Model file for the job. Use its own axes, mm. A direction names the side the tool comes from. Coordinates: 2 decimals unless noted, no trailing zeros. Order: outer loops, then holes, each group sorted by start corner. A loop starts at its lowest first (then second) coordinate and runs counter-clockwise, first axis right, second up. Notation, with made-up numbers: (-26, 87.25) -> (33, 87.25) arc R34 ccw to (33, 121.25) -> close; hole circle Ø7 at (73.5, 84). An arc over 180 degrees is marked (long way). Return JSON: item names as keys, results as strings. Group by question number.
1) Probe line 1 (X direction, y = 3.5, z = 22); line 2 (Z direction, x = -8.25, y = -1.5); line 3 (X direction, y = 3, z = 45.5). List the from-to ranges inside material, lowest first.
2) Cut at A-A (x = -14.75). Write the cut outline in (y, z) (3 decimals).
3) Flat gauge pins, fed straight in: pin 1 (3 mm diameter, centred on y = 2, z = 11.5, fed in from -X); pin 2 (1.8 mm diameter, centred on x = -15.32, z = 44.54, fed in from -Y); pin 3 (1.5 mm diameter, centred on y = 3, z = 33, fed in from +X); pin 4 (1.5 mm diameter, centred on x = -5.5, y = -2.5, fed in from +Z). Where does each tip first touch, or does it go through?
4) Pull direction Z, two halves, no side cores. Call faces 3 (the cylindrical face through (-0.56, -0.06, 2.72)), 4 (the cylindrical face through (-0.69, -0.06, 0.49)), 5 (the flat face through (-7, 4.5, 25)), 6 (the flat face through (-5.845, -0.063, 36.124)): +Z half, -Z half, draft (parallel to the pull), parting line (faces both ways), or undercut.
5) Cut at C-C (z = 45.5). Write the cut outline in (x, y), and give its area (3 significant figures).
6) Cut at D-D (z = 18.5). Write the cut outline in (x, y).
7) Cut at B-B (y = 3.5). Write the cut outline in (x, z), and give its area (3 significant figures).
8) Which spindle directions (+Z, -Z, +X, -X, +Y, -Y) get a long thin tool onto all of the face, cutting with end or side? Do faces 1 (the flat face through (-4, 0, 0)), 2 (the flat face through (-8, 0, 13)). Say none if no direction does.
Autodesk Inventor part; units mm, degrees
ref_plane "YZ Plane" through (0, 0, 0) normal (1, 0, 0) x (0, 1, 0)
ref_plane "XZ Plane" through (0, 0, 0) normal (0, 1, 0) x (-1, 0, 0)
ref_plane "XY Plane" through (0, 0, 0) normal (0, 0, 1) x (1, 0, 0)
sketch "Boceto1" plane through (0, 0, 0) normal (0, 1, 0) x (-1, 0, 0)
  line L0 (0, 2) -> (0, 26)
  line L1 (0, 26) -> (11.8564, 46.5359)
  line L2 (17.3205, 48) -> (17.3205, 48)
  line L3 (18.7846, 42.5359) -> (8, 23.8564)
  line L4 (8, 23.8564) -> (8, 2)
  line L5 (6, 0) -> (2, 0)
  arc A0 (81.7987, 0) -> (84.2987, 9.3301) centre (81.7987, 5) ccw
  arc A1 (18.7846, 42.5359) -> (17.3205, 48) centre (15.3205, 44.5359) ccw
  arc A2 (17.3205, 48) -> (11.8564, 46.5359) centre (15.3205, 44.5359) ccw
  arc A3 (6, 0) -> (8, 2) centre (6, 2) ccw
  arc A4 (0, 2) -> (2, 0) centre (2, 2) ccw
  circle A5 centre (15.3205, 44.5359) radius 1.5
  line L6 (15.3205, 44.5359) -> (4.5694, 25.9145) construction
  circle A6 centre (8.3205, 32.4115) radius 1.5
  point P0 (0, 0)
  point P1 (13.8564, 50)
  point P2 (8, 0)
  point P3 (20.7846, 46)
  point P4 (4, 0)
  dimension "d0" = 90
  dimension "d2" = 26
  dimension "d7" = 8
  dimension "d10" = 150
  dimension "d11" = 8
  dimension "d12" = 5
  dimension "d13" = 4
  dimension "d14" = 4
  dimension "d15" = 2
  dimension "d16" = 3
  dimension "d17" = 3
  dimension "d18" = 14
  dimension "d19" = 48
extrude "Extrusión1" add sketch "Boceto1" along normal mid plane 9
sketch "Boceto2" plane through (0, -4.5, 0) normal (0, -1, 0) x (1, 0, 0)
  arc A0 (-1.5, 18.0359) -> (-1.5, 21.0359) centre (-1.5, 19.5359) ccw
  arc A1 (-1.5, 18.0359) -> (-1.5, 15.0359) centre (-1.5, 16.5359) ccw
  arc A2 (-1.5, 12.0359) -> (-1.5, 15.0359) centre (-1.5, 13.5359) ccw
  arc A3 (-2, 0) -> (0, 2) centre (-2, 2) ccw construction
  arc A4 (-1.5, 12.0359) -> (-1.5, 9.0359) centre (-1.5, 10.5359) ccw
  arc A5 (-1.5, 6.0359) -> (-1.5, 9.0359) centre (-1.5, 7.5359) ccw
  arc A6 (-1.5, 6.0359) -> (-1.5, 3.0359) centre (-1.5, 4.5359) ccw
  arc A7 (-1.5, 0.0523) -> (-1.6566, 3.0441) centre (-1.5, 1.5523) ccw
  line L0 (-1.5, 31) -> (-1.5, -6.4684) construction
  line L1 (0, 26) -> (0, 2) construction
  line L2 (0, 1.5523) -> (0, 19.5359)
  point P0 (0, 0)
  point P1 (0, 7.5359)
  point P2 (0, 13.5359)
  dimension "d24" = 3
  dimension "d25" = 3
  dimension "d26" = 3
  dimension "d27" = 3
  dimension "d28" = 3
  dimension "d29" = 3
  dimension "d30" = 3
  dimension "d31" = 1.5
extrude "Extrusión2" cut sketch "Boceto2" against normal blind 9
equation "\"Radio_pliegue\" = Grosor"
equation "\"Anchura_desahogo_plegado\" = Grosor"
equation "\"Profundidad_desahogo_plegado\" = 0.5 * Grosor"
equation "\"Tamaño_destalonado\" = 4 * Grosor"
equation "\"Remanente_mínimo\" = 2 * Grosor"
equation "\"Radiodetransición\" = Radio_pliegue"
equation "\"Tamaño_de_radio_de_Jacobi\" = Radio_pliegue"
equation "\"TamañoSeparación\" = Grosor"
properties part number "Pinza_pieza3"
Answers below:
{
 "1": {"line 1": "x = -8 to 0", "line 2": "z = 24.29 to 30.91, 33.91 to 40.29", "line 3": "x = -19.2 to -16.47, -14.17 to -11.26"},
 "2": {"outline": "(-4.5, 35.548) -> (4.5, 35.548) -> (4.5, 43.149) -> (-4.5, 43.149) -> close; (-4.5, 45.923) -> (4.5, 45.923) -> (4.5, 48.495) -> (-4.5, 48.495) -> close"},
 "3": {"pin 1": "stops at x = -8", "pin 2": "passes through", "pin 3": "stops at x = -3.61", "pin 4": "stops at z = 36.83"},
 "4": {"face 3": "undercut", "face 4": "-Z half", "face 5": "draft", "face 6": "+Z half"},
 "5": {"outline": "(-19.2, -4.5) -> (-16.47, -4.5) -> (-16.47, 4.5) -> (-19.2, 4.5) -> close; (-14.17, -4.5) -> (-11.26, -4.5) -> (-11.26, 4.5) -> (-14.17, 4.5) -> close", "area": "50.8 mm^2"},
 "6": {"outline": "(-8, -4.5) -> (-0.42, -4.5) -> (-0.42, 4.5) -> (-8, 4.5) -> close"},
 "7": {"outline": "(-18.78, 42.54) -> (-8, 23.86) -> (-8, 2) arc R2 ccw to (-6, 0) -> (-2, 0) arc R2 ccw to (-0.01, 1.76) arc R1.5 ccw to (-1.66, 3.04) arc R1.5 cw to (-1.5, 6.04) arc R1.5 ccw to (-1.5, 9.04) arc R1.5 cw to (-1.5, 12.04) arc R1.5 ccw to (-1.5, 15.04) arc R1.5 cw to (-1.5, 18.04) arc R1.5 ccw to (0, 19.54) -> (0, 26) -> (-11.86, 46.54) arc R4 ccw to start; hole circle Ø3 at (-15.32, 44.54); hole circle Ø3 at (-8.32, 32.41)", "area": "363 mm^2"},
 "8": {"face 1": "-Z, +X, -X, +Y, -Y", "face 2": "-Z, -X, +Y, -Y"}
}
